Part model, mm, in its own coordinate system. Give positions to 0.01 mm unless a question says otherwise; leave off trailing zeros. Loops run counter-clockwise (first coordinate to the right, second up) from the corner with the lowest first, then second, coordinate; pieces in that order, holes last. Notation, with made-up numbers: M 83,-18 L 109,-18 A37 ccw 109,21 Z; hole C 5,9.25 d2. An arc over 180 degrees is marked long. Answer in a Markdown table with one row per item.
from build123d import *

# Parameters (mm, degrees)
F1_DEPTH = 800
F2_R     = 3
F3_DEPTH = 25
F5_R     = 6
F6_DEPTH = 40.001


with BuildPart() as f1:
    # F0 (on Top) → F1 (new body)
    with BuildSketch(Plane.XY):
        with BuildLine():
            Line((-15, -20), (15, -20))
            ThreePointArc((15, -20), (18.535534, -18.535534), (20, -15))
            Line((20, -15), (20, 15))
            ThreePointArc((20, 15), (18.535534, 18.535534), (15, 20))
            Line((15, 20), (-15, 20))
            ThreePointArc((-15, 20), (-18.535534, 18.535534), (-20, 15))
            Line((-20, 15), (-20, -15))
            ThreePointArc((-20, -15), (-18.535534, -18.535534), (-15, -20))
        make_face()
        with BuildLine():
            ThreePointArc((18, -15), (17.12132, -17.12132), (15, -18))
            Line((15, -18), (-15, -18))
            ThreePointArc((-15, -18), (-17.12132, -17.12132), (-18, -15))
            Line((-18, -15), (-18, 15))
            ThreePointArc((-18, 15), (-17.12132, 17.12132), (-15, 18))
            Line((-15, 18), (15, 18))
            ThreePointArc((15, 18), (17.12132, 17.12132), (18, 15))
            Line((18, 15), (18, -15))
        make_face(mode=Mode.SUBTRACT)
    extrude(amount=F1_DEPTH)

    # F2 (on face) → F3 (cut)
    with BuildSketch(Plane.XZ.offset(20)):
        with Locations((0, 775)):
            Circle(F2_R)
        with Locations((0, 735)):
            Circle(F2_R)
    extrude(amount=-F3_DEPTH, mode=Mode.SUBTRACT)

    # F5 (on face) → F6 (cut, through all)
    with BuildSketch(Plane.XZ.offset(20)):
        with Locations((0, 455)):
            Circle(F5_R)
        with Locations((0, 30)):
            Circle(F5_R)
    extrude(amount=-F6_DEPTH, mode=Mode.SUBTRACT)


solid = f1.part
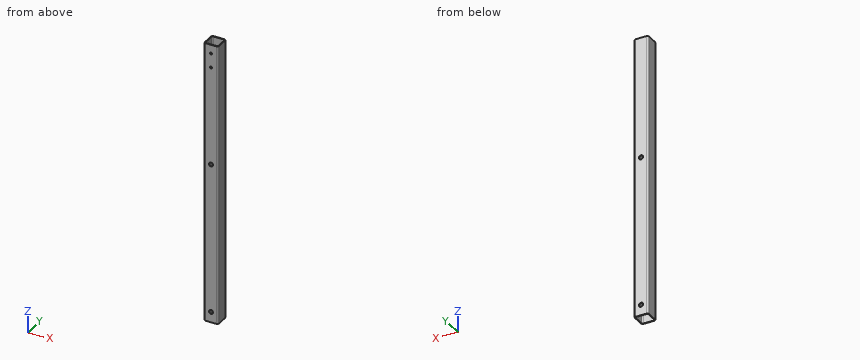
(1) Pin check, flat tips, straight feed: pin 1 Ø1 at (y, z) = (15.5, 586) entering from -X; pin 2 Ø7 at (x, z) = (0, 455) entering from -Y. Stop position of each tip, or through.
Recorded:
| item | result |
|---|---|
| pin 1 | stops at x = -20 |
| pin 2 | passes through |
(2) Drill centre lines: line 1 along Z through (x, y) = (0, -18.85); line 2 along Z through (x, y) = (0, 18.9); line 3 along X through (y, z) = (-19, 775). Where is each one in solid material? Low to high.
Recorded:
| item | result |
|---|---|
| line 1 | z = 0 to 24, 36 to 449, 461 to 732, 738 to 772, 778 to 800 |
| line 2 | z = 0 to 24, 36 to 449, 461 to 800 |
| line 3 | x = -18 to -3, 3 to 18 |
(3) Saw through at B-B (z = 633). Write the cut outline in (x, y).
Recorded:
| item | result |
|---|---|
| outline | M -20,-15 A5 ccw -15,-20 L 15,-20 A5 ccw 20,-15 L 20,15 A5 ccw 15,20 L -15,20 A5 ccw -20,15 Z; hole M -18,-15 A3 ccw -15,-18 L 15,-18 A3 ccw 18,-15 L 18,15 A3 ccw 15,18 L -15,18 A3 ccw -18,15 Z |
(4) Saw through at A-A (y = -6.5). Write the cut outline in (x, z).
Recorded:
| item | result |
|---|---|
| outline | M -20,0 L -18,0 L -18,800 L -20,800 Z; M 18,0 L 20,0 L 20,800 L 18,800 Z |
